Autodesk Fusion 360 part; units mm, degrees
sketch "Szkic1" plane through (0, 0, 0) normal (0, 0, 1) x (1, 0, 0)
  line L0 (-20, 25) -> (-20, -25)
  line L1 (-20, -25) -> (0, -25)
  line L2 (0, -25) -> (0, 25)
  line L3 (0, 25) -> (-20, 25)
  line L4 (0, 10) -> (0, -10)
  line L5 (0, -10) -> (20, -10)
  line L6 (20, -10) -> (20, 10)
  line L7 (20, 10) -> (0, 10)
  circle A0 centre (10, 0) radius 3
  circle A1 centre (10, 0) radius 5.5
  line L8 (-12.5, 25) -> (-7.5, 25)
  line L9 (-7.5, 25) -> (-7.5, -25)
  line L10 (-7.5, -25) -> (-12.5, -25)
  line L11 (-12.5, -25) -> (-12.5, 25)
  dimension "d1" = 6
  dimension "d2" = 11
extrude "Wyciągnięcie proste1" add sketch "Szkic1" against normal blind 25 contours L0 L1 L3 L11 | L1 L3 L8 L9 L10 L11 | L1 L2 L3 L4 L9 | L2 L4 L5 L6 L7
extrude "Wyciągnięcie proste2" add sketch "Szkic1" against normal blind 4.2 contours A0 | A1
extrude "Wyciągnięcie proste3" cut sketch "Szkic1" against normal blind 4 contours A0
extrude "Wyciągnięcie proste4" add sketch "Szkic1" along normal blind 5 contours L1 L3 L8 L9 L10 L11
chamfer "Fazowanie1" distance 5 angle 45 1 edges at (0, -10, -12.5)
chamfer "Fazowanie2" distance 5 angle 45 1 edges at (0, 10, -12.5)
chamfer "Fazowanie3" distance 3 angle 45 6 edges at (20, 10, -12.5) (20, -10, -12.5) (0, 25, -12.5) (-20, 25, -12.5) (-20, -25, -12.5) (0, -25, -12.5)
chamfer "Fazowanie4" distance 1 angle 45 1 faces at (-11.8333, 0, -25)
delete_face "Usuń powierzchnię1" 1 faces at (16.159, -0.3074, -24.6667)
Can you work these out from the model? Positions are in its coordinate system, mm. A direction names the side the tool comes from. Round coordinates to 2 decimals unless told otherwise and drop trailing zeros. Write each loop counter-clockwise with the first axis right and the second up, starting at its lowest first coordinate (ties: lowest second). Pieces come first, ordered by that corner, then holes. Notation, with made-up numbers: (72.25, 38.5) -> (76.25, 38.5) arc R18 ccw to (76.25, 61.5) -> close; hole circle Ø1 at (3.25, 74). An arc over 180 degrees is marked (long way). Use one line per item in the form item = value. Start each with the question number.
Q1. We'd pull the mould along X, two halves only. Please class faces 1 (the face through (-2, 24, -12)), 2 (the face through (15.08, -2.11, -14.45)), 3 (the face through (12.77, -1.15, -1.97)), 4 (the face through (-19, 23, -12)): +X half, -X half, draft (parallel to the pull), parting line (faces both ways), or undercut.
Q2. Which directions (+Z, -Z, +X, -X, +Y, -Y) give clear straight access to the entire face, cutting with the end or side of a thin tool? Please do faces 5 (the face through (-16, 0, 0)), 6 (the face through (11, -10, -12)), 7 (the face through (-4, 0, -25)), 8 (the face through (0, 18, -12)).
Q3. Imagine slicing it at A-A (z = -5). Please give me the cut outline in (x, y).
Q4. Imagine slicing it at C-C (x = 10). Please give me the cut outline in (y, z).
Q5. If I drill on probe 1 along Y at (x, z) = (10, -2); probe 2 along Y at (x, z) = (10, -17); probe 3 along Z at (x, y) = (-1.5, 4), over which ranges is the centre line in solid material (lowest first)? Write a range as [from, to].
Q6. Imagine slicing it at B-B (y = 0). Please give me the cut outline in (x, z), then the cut area to 3 significant figures.
Q7. I'm going to push flat-ended pins straight in: P1, Ø5, axis at x = 10, y = 1, coming from the +Z side; P2, Ø6, axis at x = 10, z = -14.5, coming from the -Y side; P3, Ø4, axis at y = 18.5, z = -4, coming from the +X side; P4, Ø2, axis at x = 3, y = 14.5, coming from the -Z side. Where does each tip first touch, or does it pass through?
Q8. Imagine slicing it at D-D (y = 20.5). Please give me the cut outline in (x, z).
Worked out:
q1.face_1 = +X half
q1.face_2 = undercut
q1.face_3 = undercut
q1.face_4 = -X half
q2.face_5 = +Z, -X, +Y, -Y
q2.face_6 = +Z, -Z, +X, -Y
q2.face_7 = -Z, +X, -X, +Y, -Y
q2.face_8 = +Z, -Z, +X, +Y
q3.outline = (-20, -22) -> (-17, -25) -> (-3, -25) -> (0, -22) -> (0, -15) -> (5, -10) -> (17, -10) -> (20, -7) -> (20, 7) -> (17, 10) -> (5, 10) -> (0, 15) -> (0, 22) -> (-3, 25) -> (-17, 25) -> (-20, 22) -> close; hole circle Ø11 at (10, 0)
q4.outline = (-10, -24) -> (-9, -25) -> (-5.5, -25) -> (-5.5, -4.2) -> (5.5, -4.2) -> (5.5, -25) -> (9, -25) -> (10, -24) -> (10, 0) -> (3, 0) -> (3, -4) -> (-3, -4) -> (-3, 0) -> (-10, 0) -> close
q5.probe_1 = [-10, -3], [3, 10]
q5.probe_2 = [-10, -5.5], [5.5, 10]
q5.probe_3 = [-25, 0]
q6.outline = (-20, -24) -> (-19, -25) -> (4.5, -25) -> (4.5, -4.2) -> (15.5, -4.2) -> (15.5, -25) -> (19, -25) -> (20, -24) -> (20, 0) -> (13, 0) -> (13, -4) -> (7, -4) -> (7, 0) -> (-7.5, 0) -> (-7.5, 5) -> (-12.5, 5) -> (-12.5, 0) -> (-20, 0) -> close
q6.area = 771 mm^2
q7.P1 = 0
q7.P2 = -10
q7.P3 = 0
q7.P4 = through
q8.outline = (-20, -24) -> (-19, -25) -> (-1, -25) -> (0, -24) -> (0, 0) -> (-7.5, 0) -> (-7.5, 5) -> (-12.5, 5) -> (-12.5, 0) -> (-20, 0) -> close
